```python
from build123d import *

# Parameters (mm, degrees)
SALIENTE_EXTRUIR1_DEPTH = 205
CORTAR_EXTRUIR1_REACH   = 211.458
CROQUIS2_R              = 3
CHAFL_N1_SIZE           = 0.5
CROQUIS3_W              = 43.76
CROQUIS3_H              = 18.5
CORTAR_EXTRUIR2_DEPTH   = 210.458192487


with BuildPart() as part:
    # Croquis1 → Saliente-Extruir1 (new, symmetric)
    with BuildSketch(Plane.XY):
        with BuildLine():
            Line((-8.121192263, 10), (-3.67559519, 17.7))
            ThreePointArc((-3.67559519, 17.7), (0, 37), (3.67559519, 17.7))
            Line((3.67559519, 17.7), (8.121192263, 10))
            Line((8.121192263, 10), (9.5, 10))
            Line((9.5, 10), (9.5, 5))
            Line((9.5, 5), (21.88, 5))
            Line((21.88, 5), (21.88, 0))
            Line((21.88, 0), (-21.88, 0))
            Line((-21.88, 0), (-21.88, 5))
            Line((-21.88, 5), (-9.5, 5))
            Line((-9.5, 5), (-9.5, 10))
            Line((-9.5, 10), (-8.121192263, 10))
        make_face()
    extrude(amount=SALIENTE_EXTRUIR1_DEPTH, both=True)

    # Croquis2 → Cortar-Extruir1 (cut, up to next)
    with BuildSketch(Plane.XZ, mode=Mode.PRIVATE) as cortar_extruir1_sk1:
        with Locations(Location((15, 150, 0), (0, 0, 270))):
            Circle(CROQUIS2_R)
    cortar_extruir1_tool1 = extrude(cortar_extruir1_sk1.sketch, amount=-CORTAR_EXTRUIR1_REACH, mode=Mode.PRIVATE) & part.part
    # Croquis2 → Cortar-Extruir1 (cut, up to next)
    with BuildSketch(Plane.XZ, mode=Mode.PRIVATE) as cortar_extruir1_sk2:
        with Locations(Location((-15, 150, 0), (0, 0, 270))):
            Circle(CROQUIS2_R)
    cortar_extruir1_tool2 = extrude(cortar_extruir1_sk2.sketch, amount=-CORTAR_EXTRUIR1_REACH, mode=Mode.PRIVATE) & part.part
    # Croquis2 → Cortar-Extruir1 (cut, up to next)
    with BuildSketch(Plane.XZ, mode=Mode.PRIVATE) as cortar_extruir1_sk3:
        with Locations(Location((-15, 0, 0), (0, 0, 270))):
            Circle(CROQUIS2_R)
    cortar_extruir1_tool3 = extrude(cortar_extruir1_sk3.sketch, amount=-CORTAR_EXTRUIR1_REACH, mode=Mode.PRIVATE) & part.part
    # Croquis2 → Cortar-Extruir1 (cut, up to next)
    with BuildSketch(Plane.XZ, mode=Mode.PRIVATE) as cortar_extruir1_sk4:
        with Locations(Location((15, 0, 0), (0, 0, 270))):
            Circle(CROQUIS2_R)
    cortar_extruir1_tool4 = extrude(cortar_extruir1_sk4.sketch, amount=-CORTAR_EXTRUIR1_REACH, mode=Mode.PRIVATE) & part.part
    # Croquis2 → Cortar-Extruir1 (cut, up to next)
    with BuildSketch(Plane.XZ, mode=Mode.PRIVATE) as cortar_extruir1_sk5:
        with Locations(Location((15, -150, 0), (0, 0, 270))):
            Circle(CROQUIS2_R)
    cortar_extruir1_tool5 = extrude(cortar_extruir1_sk5.sketch, amount=-CORTAR_EXTRUIR1_REACH, mode=Mode.PRIVATE) & part.part
    # Croquis2 → Cortar-Extruir1 (cut, up to next)
    with BuildSketch(Plane.XZ, mode=Mode.PRIVATE) as cortar_extruir1_sk6:
        with Locations(Location((-15, -150, 0), (0, 0, 270))):
            Circle(CROQUIS2_R)
    cortar_extruir1_tool6 = extrude(cortar_extruir1_sk6.sketch, amount=-CORTAR_EXTRUIR1_REACH, mode=Mode.PRIVATE) & part.part
    add(cortar_extruir1_tool1.solids().sort_by_distance((15, 0, 150))[0], mode=Mode.SUBTRACT)
    add(cortar_extruir1_tool2.solids().sort_by_distance((-15, 0, 150))[0], mode=Mode.SUBTRACT)
    add(cortar_extruir1_tool3.solids().sort_by_distance((-15, 0, 0))[0], mode=Mode.SUBTRACT)
    add(cortar_extruir1_tool4.solids().sort_by_distance((15, 0, 0))[0], mode=Mode.SUBTRACT)
    add(cortar_extruir1_tool5.solids().sort_by_distance((15, 0, -150))[0], mode=Mode.SUBTRACT)
    add(cortar_extruir1_tool6.solids().sort_by_distance((-15, 0, -150))[0], mode=Mode.SUBTRACT)

    # Chaflán1
    chafl_n1_edges = [part.edges().sort_by_distance(p)[0] for p in [
        (-15, 5, 153),
        (-15, 5, 3),
        (15, 5, 3),
        (15, 5, -147),
        (-15, 5, -147),
        (15, 5, 153),
    ]]
    chamfer(chafl_n1_edges, length=CHAFL_N1_SIZE)

    # Croquis3 → Cortar-Extruir2 (cut, through all)
    with BuildSketch(Plane.XZ):
        with Locations((0, -195.75)):
            Rectangle(CROQUIS3_W, CROQUIS3_H)
    extrude(amount=-CORTAR_EXTRUIR2_DEPTH, mode=Mode.SUBTRACT)


solid = part.part
```
Geometry: final body of the model. Coordinates: model frame, mm. Round coordinates to 2 decimals unless told otherwise and drop trailing zeros. Loops run counter-clockwise (first coordinate to the right, second up) from the corner with the lowest first, then second, coordinate; pieces in that order, holes last.
Item 1: Section B-B, the plane y = 28.5. Output: boundary loops of the cut face in (x, z).
Checked values:
outline: (-9.89, -186.5) - (9.89, -186.5) - (9.89, 205) - (-9.89, 205) - close
Item 2: Section A-A, the plane z = -100. Output: boundary loops of the cut face in (x, y), plus the area to 3 significant figures.
Checked values:
outline: (-21.88, 0) - (21.88, 0) - (21.88, 5) - (9.5, 5) - (9.5, 10) - (8.12, 10) - (3.68, 17.7) arc R10 ccw (long way) to (-3.68, 17.7) - (-8.12, 10) - (-9.5, 10) - (-9.5, 5) - (-21.88, 5) - close
area: 715 mm2
Item 3: Mould query, pull axis X, two halves, no side actions, for faces 1 (the cylindrical face through (13.85, 2.22, 147.23)), 2 (the flat face through (5.87, 13.9, 11.99)), 3 (the flat face through (-5.93, 13.796, 11.99)), 4 (the flat face through (16, 5, 12)). Classes: released by +X, released by -X, zero draft, split by the parting line, or undercut.
Checked values:
face 1: undercut
face 2: released by +X
face 3: released by -X
face 4: zero draft
Item 4: Line query: L1, parallel to X at y = 1.85, z = 0; L2, parallel to Z at x = 15.5, y = 2; L3, parallel to Y at x = -17, z = 90. Output: solid intervals per line, ascending.
Checked values:
L1: x = -21.88 to -18, -12 to 12, 18 to 21.88
L2: z = -186.5 to -152.96, -147.04 to -2.96, 2.96 to 147.04, 152.96 to 205
L3: y = 0 to 5
Item 5: Contact query for flat-ended pins moving along their axis: P1, Ø8, axis at x = -15, z = -150, coming from the +Y side; P2, Ø3.5, axis at x = 15, z = 0, coming from the +Y side; P3, Ø5.5, axis at y = 8, z = 51.5, coming from the -X side; P4, Ø0.7, axis at x = -8.5, z = 53.5, coming from the +Y side. Output: stop coordinate, or through.
Checked values:
P1: stops at y = 5
P2: passes through
P3: stops at x = -9.5
P4: stops at y = 32.79
